```python
from build123d import *

# Parameters (mm, degrees)
SKETCH_1_W          = 600
SKETCH_1_H          = 455
EXTRUDE_1_DEPTH     = 195
LOFT_1_OUTLINE_W    = 360
LOFT_1_OUTLINE_H    = 215
LOFT_1_DEPTH        = 170
LOFT_1_DRAFT        = -6.7098368
SHELL_1_T           = -20
SKETCH_3_R          = 25
SKETCH_3_R_2        = 17.5
CUT_EXTRUDE_2_DEPTH = 777.61122835
FILLET_1_R          = 10


# Read off the part's stored shape, not the designer's step: Вырез-По сечениям1
with BuildPart() as part:
    # Эскиз1 → Бобышка-Вытянуть1 (new body)
    with BuildSketch(Plane(origin=(0, 0, 0), x_dir=(1, 0, 0), z_dir=(0, 1, 0))):
        with Locations((300, 227.5)):
            Rectangle(SKETCH_1_W, SKETCH_1_H)
    extrude(amount=EXTRUDE_1_DEPTH)


with BuildPart() as loft_1_tool:
    # Вырез-По сечениям1 outline → Вырез-По сечениям1 (with draft: the straight prism first)
    with BuildSketch(Plane(origin=(0, 25, 0), x_dir=(1, 0, 0), z_dir=(0, 1, 0))):
        with Locations((300, 227.5)):
            Rectangle(LOFT_1_OUTLINE_W, LOFT_1_OUTLINE_H)
    extrude(amount=LOFT_1_DEPTH)
    # Вырез-По сечениям1: the draft: its side faces are tilted about the plane it starts from
    loft_1_sides = [loft_1_tool.faces().sort_by_distance(p)[0] for p in [
        (480, 110, -227.5),
        (300, 110, -335),
        (120, 110, -227.5),
        (300, 110, -120),
    ]]
    draft(loft_1_sides, Plane(origin=(0, 25, 0), x_dir=(1, 0, 0), z_dir=(0, 1, 0)), LOFT_1_DRAFT)


with BuildPart() as part_1:
    add(part.part)

    # Вырез-По сечениям1: cut by loft_1_tool
    add(loft_1_tool.part, mode=Mode.SUBTRACT)

    # Оболочка1
    shell_1_openings = [part_1.faces().sort_by_distance(p)[0] for p in [
        (300, 97.5, 0),
        (0, 97.5, -227.5),
        (600, 97.5, -227.5),
        (300, 0, -227.5),
        (300, 97.5, -455),
    ]]
    offset(amount=SHELL_1_T, openings=shell_1_openings, kind=Kind.INTERSECTION)

    # Эскиз3 → Вырез-Вытянуть2 (cut, through all)
    with BuildSketch(Plane(origin=(0, 195, 0), x_dir=(-1, 0, 0), z_dir=(0, 1, 0))):
        with Locations(Location((-300, -255, 0), (0, 0, 90))):
            Circle(SKETCH_3_R)
        with Locations(Location((-300, -405, 0), (0, 0, 90))):
            Circle(SKETCH_3_R_2)
    extrude(amount=-CUT_EXTRUDE_2_DEPTH, mode=Mode.SUBTRACT)

    # Скругление1
    fillet_1_edges = [part_1.edges().sort_by_distance(p)[0] for p in [
        (300, 195, -455),
        (600, 195, -227.5),
        (300, 195, 0),
        (0, 195, -227.5),
        (100.000000023, 195, -227.5),
        (300, 195, -100.000000023),
        (499.999999977, 195, -227.5),
        (300, 195, -422.5),
        (110.000000012, 110, -344.999999988),
        (300, 195, -354.999999977),
        (489.999999988, 110, -344.999999988),
        (300, 25, -120),
        (120, 25, -227.5),
        (300, 25, -335),
        (480, 25, -227.5),
        (300, 25, -280),
    ]]
    fillet(fillet_1_edges, radius=FILLET_1_R)


solid = part_1.part
```
Input: part model. Units: mm. Frame: model coordinates. A direction names the side the tool comes from. Give positions to 0.01 mm unless a question says otherwise; leave off trailing zeros. Loops run counter-clockwise (first coordinate to the right, second up) from the corner with the lowest first, then second, coordinate; pieces in that order, holes last. Notation, with made-up numbers: (-4.5, 3) -> (44.5, 3) arc R35 cw to (44.5, 42) -> close; hole circle Ø1 at (79, 8.5). An arc over 180 degrees is marked (long way). Use a Markdown table: item, result.
Q1. Access query for faces 5 (the cylindrical face through (307.509, 10.07, -231.154)), 6 (the cylindrical face through (487.309, 111.132, -342.155)). Directions: +Z, -Z, +X, -X, +Y, -Y. A direction counts if a zero-diameter tool reaches every point of the face in a straight line with its end or side. Return the directions, or none.
Entries:
| item | result |
|---|---|
| face 5 | +Y, -Y |
| face 6 | +Y |
Q2. Pull-direction query (X, two-part tool) for faces 1 (the flat face through (507.645, 88.81, -225.466)), 2 (the flat face through (296.951, 88.81, -92.355)), 3 (the flat face through (297.215, 108.934, -110.125)), 4 (the flat face through (298, 25, -207)); classes: pulls with the +X half, pulls with the -X half, needs draft (parallel to the pull), parting line crosses it, or undercut.
Entries:
| item | result |
|---|---|
| face 1 | pulls with the +X half |
| face 2 | needs draft |
| face 3 | undercut |
| face 4 | undercut |
Q3. First-contact query: P1, Ø10, axis at y = 125, z = -211, coming from the +X side; P2, Ø10, axis at y = 142.5, z = -92, coming from the +X side; P3, Ø3, axis at y = 139, z = -116.5, coming from the +X side. Flat tips, straight axial feed; report the tip coordinate or a pass-through.
Entries:
| item | result |
|---|---|
| P1 | stops at x = 512.49 |
| P2 | stops at x = 514.55 |
| P3 | stops at x = 513.73 |
Q4. Section query C-C, the plane z = -142.5. Return the cut outline in (x, y) (1 decimal).
Entries:
| item | result |
|---|---|
| outline | (0, 175) -> (82.2, 175) -> (102.2, 5) -> (497.8, 5) -> (517.8, 175) -> (600, 175) -> (600, 185) arc R10 ccw to (590, 195) -> (508.9, 195) arc R10 ccw to (499, 186.2) -> (481, 33.8) arc R10 cw to (471.1, 25) -> (128.9, 25) arc R10 cw to (119, 33.8) -> (101, 186.2) arc R10 ccw to (91.1, 195) -> (10, 195) arc R10 ccw to (0, 185) -> close |
Q5. Section query A-A, the plane z = -405. Return the cut outline in (x, y).
Entries:
| item | result |
|---|---|
| outline | (0, 175) -> (282.5, 175) -> (282.5, 185) arc R10 ccw to (272.5, 195) -> (10, 195) arc R10 ccw to (0, 185) -> close; (317.5, 175) -> (600, 175) -> (600, 185) arc R10 ccw to (590, 195) -> (327.5, 195) arc R10 ccw to (317.5, 185) -> close |
Q6. Section query B-B, the plane x = 300. State how many separate pieces and enclosed holes the cut face has, plus the area to 3 significant figures.
Entries:
| item | result |
|---|---|
| separate pieces | 3 |
| enclosed holes | 0 |
| area | 13,300 mm² |
Q7. Ray query, probe 1 along X at (y, z) = (179, -405); probe 2 along Y at (x, z) = (60, -200); probe 3 along X at (y, z) = (127, -303). Return the intervals inside material, ascending. Write a range as from..to.
Entries:
| item | result |
|---|---|
| probe 1 | x = 0..282.5, 317.5..600 |
| probe 2 | y = 175..195 |
| probe 3 | x = 87.86..108, 492..512.14 |
Q8. Section query D-D, the plane x = 449. Return the cut outline in (y, z) (1 decimal).
Entries:
| item | result |
|---|---|
| outline | (5, -352.8) -> (175, -372.8) -> (175, -455) -> (185, -455) arc R10 ccw to (195, -445) -> (195, -363.9) arc R10 ccw to (186.2, -354) -> (33.8, -336) arc R10 cw to (25, -326.1) -> (25, -128.9) arc R10 cw to (33.8, -119) -> (186.2, -101) arc R10 ccw to (195, -91.1) -> (195, -10) arc R10 ccw to (185, 0) -> (175, 0) -> (175, -82.2) -> (5, -102.2) -> close |
